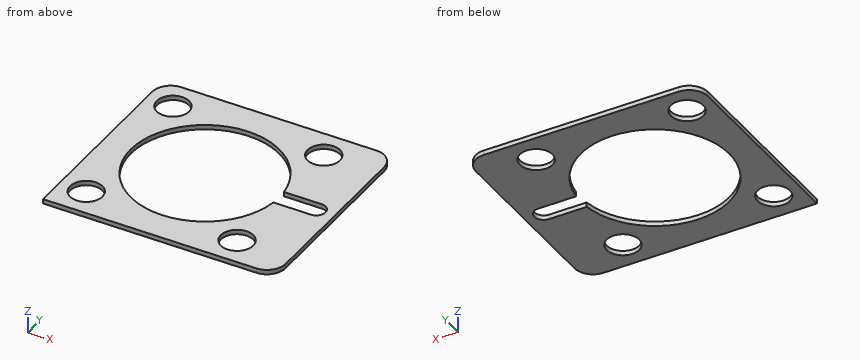
Autodesk Inventor part; units mm, degrees
ref_plane "YZ Plane" through (0, 0, 0) normal (1, 0, 0) x (0, 1, 0)
ref_plane "XZ Plane" through (0, 0, 0) normal (0, 1, 0) x (-1, 0, 0)
ref_plane "XY Plane" through (0, 0, 0) normal (0, 0, 1) x (1, 0, 0)
sketch "Sketch1" plane through (0, 0, 0) normal (0, 0, 1) x (1, 0, 0)
  line L0 (-45.72, 57.15) -> (60.96, 57.15)
  line L1 (71.12, 46.99) -> (71.12, -46.99)
  line L2 (60.96, -57.15) -> (-55.88, -57.15)
  line L3 (-55.88, -57.15) -> (-55.88, 46.99)
  line L4 (-84.7488, 0) -> (99.553, 0)
  line L5 (0, -82.9559) -> (0, 82.9559)
  arc A0 (40.3212, 5.08) -> (40.3212, -5.08) centre (0, 0) ccw
  circle A1 centre (0, 0) radius 58.42 construction
  arc A2 (-45.72, 57.15) -> (-55.88, 46.99) centre (-45.72, 46.99) ccw
  arc A3 (71.12, 46.99) -> (60.96, 57.15) centre (60.96, 46.99) ccw
  arc A4 (60.96, -57.15) -> (71.12, -46.99) centre (60.96, -46.99) ccw
  line L6 (0, 0) -> (-50.4247, 50.4247) construction
  circle A5 centre (-41.3092, 41.3092) radius 8.89
  line L7 (0, 0) -> (-50.4247, -50.4247) construction
  circle A6 centre (-41.3092, -41.3092) radius 8.89
  line L8 (0, 0) -> (50.4247, -50.4247) construction
  circle A7 centre (41.3092, -41.3092) radius 8.89
  line L9 (0, 0) -> (50.4247, 50.4247) construction
  circle A8 centre (41.3092, 41.3092) radius 8.89
  arc A9 (60.96, -5.08) -> (60.96, 5.08) centre (60.96, 0) ccw
  line L10 (40.3212, 5.08) -> (60.96, 5.08)
  line L11 (40.3212, -5.08) -> (60.96, -5.08)
  point P0 (71.12, -57.15)
  point P1 (71.12, 57.15)
  point P2 (71.12, 0)
  dimension "d4" = 116.84
  dimension "d0" = 127
  dimension "d1" = 114.3
  dimension "d2" = 55.88
  dimension "d3" = 81.28
  dimension "d5" = 10.16
  dimension "d6" = 45
  dimension "d7" = 17.78
  dimension "d10" = 360
  dimension "d12" = 10.16
  dimension "d13" = 10.16
  dimension "d14" = 60.96
extrude "Extrusion1" add sketch "Sketch1" along normal blind 2.54 contours L0 L5 A0 L4 L3 A2 | L0 A3 L1 L4 A9 L10 A0 L5 | L4 A0 L5 L2 L3 | L1 A4 L2 L5 A0 L11 A9 L4
equation "\"BendRadius\" = Thickness"
equation "\"BendReliefWidth\" = Thickness"
equation "\"BendReliefDepth\" = 0.5 * Thickness"
equation "\"CornerReliefSize\" = 4 * Thickness"
equation "\"MinimumRemnant\" = 2 * Thickness"
equation "\"TransitionRadius\" = BendRadius"
equation "\"JacobiRadiusSize\" = BendRadius"
equation "\"GapSize\" = Thickness"
properties part number "cylinder head gasket" material "Rubber"
Geometry check sheet. Reference: the model listing, model coordinates, mm. Give positions to 0.01 mm unless a question says otherwise; leave off trailing zeros. Write each loop counter-clockwise with the first axis right and the second up, starting at its lowest first coordinate (ties: lowest second). Pieces come first, ordered by that corner, then holes.
1) Material ranges on L1, parallel to X at y = 0, z = 1.25; L2, parallel to Y at x = -1.5, z = 2.35; L3, parallel to Y at x = -44, z = 0.9, recorded low to high.
2) Section check D-D, the plane z = 0.95. Record the boundary of the cut face in (x, y), and give its area (3 significant figures).
3) Gauge pin test, flat end, axial feed: pin 1 (23 mm diameter, centred on x = -41.31, y = -41.31, fed in from +Z). Record the tip position at first contact, or that the pin passes through.
4) Section check A-A, the plane x = 0. Record the boundary of the cut face in (y, z).
5) Section check C-C, the plane y = -44. Record the boundary of the cut face in (x, z), and give its area (3 significant figures).
6) Section check B-B, the plane y = 0. Record the boundary of the cut face in (x, z).
Computed:
1. L1: x = -55.88 to -40.64, 66.04 to 71.12
1. L2: y = -57.15 to -40.61, 40.61 to 57.15
1. L3: y = -57.15 to -49.78, -32.84 to 32.84, 49.78 to 57.15
2. outline: (-55.88, -57.15) - (60.96, -57.15) arc R10.16 ccw to (71.12, -46.99) - (71.12, 46.99) arc R10.16 ccw to (60.96, 57.15) - (-45.72, 57.15) arc R10.16 ccw to (-55.88, 46.99) - close; hole circle Ø17.78 at (-41.31, -41.31); hole circle Ø17.78 at (-41.31, 41.31); hole circle Ø17.78 at (41.31, -41.31); hole circle Ø17.78 at (41.31, 41.31); hole (40.32, -5.08) - (60.96, -5.08) arc R5.08 ccw to (60.96, 5.08) - (40.32, 5.08) arc R40.64 ccw (long way) to start
2. area: 8,020 mm2
3. pin 1: stops at z = 2.54
4. outline: (-57.15, 0) - (-40.64, 0) - (-40.64, 2.54) - (-57.15, 2.54) - close; (40.64, 0) - (57.15, 0) - (57.15, 2.54) - (40.64, 2.54) - close
5. outline: (-55.88, 0) - (-49.78, 0) - (-49.78, 2.54) - (-55.88, 2.54) - close; (-32.84, 0) - (32.84, 0) - (32.84, 2.54) - (-32.84, 2.54) - close; (49.78, 0) - (71.12, 0) - (71.12, 2.54) - (49.78, 2.54) - close
5. area: 236 mm2
6. outline: (-55.88, 0) - (-40.64, 0) - (-40.64, 2.54) - (-55.88, 2.54) - close; (66.04, 0) - (71.12, 0) - (71.12, 2.54) - (66.04, 2.54) - close
